Geometry: final body of the model. Coordinates: model frame, mm. Face numbers are marked on the shaded views. A direction names the side the tool comes from. Give positions to 0.01 mm unless a question says otherwise; leave off trailing zeros. Loops run counter-clockwise (first coordinate to the right, second up) from the corner with the lowest first, then second, coordinate; pieces in that order, holes last. Notation, with made-up numbers: (88, 55.5) - (107, 55.5) arc R19 cw to (107, 81.5) - close; hole circle Ø5 at (-33, 64.5). An arc over 180 degrees is marked (long way). Answer in a Markdown table with one row per item.
from build123d import *

# Parameters (mm, degrees)
CYLINDER005_R          = 6.7
CYLINDER005_DEPTH      = 40
CYLINDER061_R          = 8.7
CYLINDER061_DEPTH      = 2.2
CYLINDER062_R          = 10.75
CYLINDER062_DEPTH      = 2.2
CYLINDER019_R          = 10.7
CYLINDER019_DEPTH      = 40
CUT022_PLACEMENT_ANGLE = 90


with BuildPart() as obj1:
    # Cylinder005 → Cylinder005 (new body)
    with BuildSketch(Plane.XY):
        Circle(CYLINDER005_R)
    extrude(amount=CYLINDER005_DEPTH)


with BuildPart() as obj2:
    # Cylinder061 → Cylinder061 (new body)
    with BuildSketch(Plane.XY.offset(10.4)):
        Circle(CYLINDER061_R)
    extrude(amount=CYLINDER061_DEPTH)


with BuildPart() as obj3:
    # Cylinder062 → Cylinder062 (new body)
    with BuildSketch(Plane.XY.offset(10.4)):
        Circle(CYLINDER062_R)
    extrude(amount=CYLINDER062_DEPTH)

    # Cut: cut obj2
    add(obj2.part, mode=Mode.SUBTRACT)

    # Fusion: union obj1
    add(obj1.part)


with BuildPart() as housingoutlet:
    # Cylinder019 → Cylinder019 (new body)
    with BuildSketch(Plane.XY):
        Circle(CYLINDER019_R)
    extrude(amount=CYLINDER019_DEPTH)


with BuildPart() as toplevelpart_outletadapter:
    # Cone001 → Cone001 (revolve)
    with BuildSketch(Plane(origin=(0, 0, 19), x_dir=(1, 0, 0), z_dir=(0, -1, 0))):
        Polygon((0, 0), (11.19, 0), (10.92, 21), (0, 21), align=None)
    revolve(axis=Axis((0, 0, 19), (0, 0, 1)))

    # Fusion054: union HousingOutlet
    add(housingoutlet.part)

    # Cut022: cut obj3
    add(obj3.part, mode=Mode.SUBTRACT)


with BuildPart() as toplevelpart_outletadapter_1:
    # Cut022 placement: moved
    add(toplevelpart_outletadapter.part.moved(Location((22, 28.6, 13.15))).rotate(Axis((22, 28.6, 13.15), (-1, 0, 0)), CUT022_PLACEMENT_ANGLE))


solid = toplevelpart_outletadapter_1.part
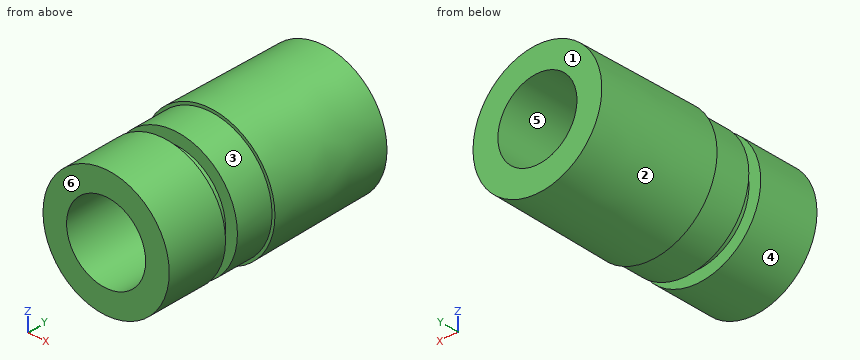
Q1. Material intervals for line 1 along X through (y, z) = (32, 13); line 2 along Y through (x, z) = (12, 12.75); line 3 along X through (y, z) = (34, 16.5), sorted ascending.
Check values:
| item | result |
|---|---|
| line 1 | 11.3 to 15.3, 28.7 to 32.7 |
| line 2 | 28.6 to 39, 41.2 to 68.6 |
| line 3 | 11.84 to 16.2, 27.8 to 32.16 |
Q2. Cut plane A-A (y = 34). Output: boundary loops of the cut face in (x, z), and give its area (3 significant figures).
Check values:
| item | result |
|---|---|
| outline | circle Ø21.4 at (22, 13.15); hole circle Ø13.4 at (22, 13.15) |
| area | 219 mm² |
Q3. First-contact query: pin 1 (1.5 mm diameter, centred on y = 58.5, z = 19.5, fed in from +X); pin 2 (12 mm diameter, centred on y = 52, z = 7, fed in from +X); pin 3 (12 mm diameter, centred on x = 22, z = 13.15, fed in from -Y); pin 4 (2 mm diameter, centred on x = 22, y = 59, fed in from -Z). Flat tips, straight axial feed; report the tip coordinate or a pass-through.
Check values:
| item | result |
|---|---|
| pin 1 | x = 31.53 |
| pin 2 | x = 33.15 |
| pin 3 | through |
| pin 4 | z = 2.09 |
Q4. Draft query along X for the marked faces 4, 5 and 6. Return one class per face: pulls with the +X half, pulls with the -X half, needs draft (parallel to the pull), parting line crosses it, or undercut.
Check values:
| item | result |
|---|---|
| face 4 | parting line crosses it |
| face 5 | undercut |
| face 6 | needs draft |
Q5. Reachability of the marked faces 1, 2 and 3 from +Z, -Z, +X, -X, +Y, -Y: full face, straight path, thin tool, end or side. Return the list, or none.
Check values:
| item | result |
|---|---|
| face 1 | +Z, -Z, +X, -X, +Y |
| face 2 | +Y |
| face 3 | -Y |
Q6. Cut plane B-B (y = 52.5). Output: boundary loops of the cut face in (x, z), and give its area (3 significant figures).
Check values:
| item | result |
|---|---|
| outline | circle Ø22.25 at (22, 13.15); hole circle Ø13.4 at (22, 13.15) |
| area | 248 mm² |
